Build history of the part. All positions in model axes, mm. A direction names the side the tool comes from. Give positions to 0.01 mm unless a question says otherwise; leave off trailing zeros. Order: outer loops, then holes, each group sorted by start corner. A loop starts at its lowest first (then second) coordinate and runs counter-clockwise, first axis right, second up. Notation, with made-up numbers: M -6.5,86.25 L -0.5,86.25 A19 cw -0.5,94.25 Z; hole C 47.25,15.25 d11. An arc over 180 degrees is marked long. One line per item, written item: value.
from build123d import *

# Parameters (mm, degrees)
F0_W     = 254
F0_H     = 127
F1_DEPTH = 76.2
F2_W     = 203.2
F2_H     = 76.2
F3_DEPTH = 152.401
F4_W     = 127
F4_H     = 55.738516
F5_DEPTH = 127.001
F6_R     = 25.4
F7_DEPTH = 254.001


with BuildPart() as f1:
    # F0 (on Top) → F1 (new body, symmetric)
    with BuildSketch(Plane.XY):
        Rectangle(F0_W, F0_H)
    extrude(amount=F1_DEPTH, both=True)

    # F2 (on face) → F3 (cut, through all)
    with BuildSketch(Plane.XY.offset(76.2)):
        Rectangle(F2_W, F2_H)
    extrude(amount=-F3_DEPTH, mode=Mode.SUBTRACT)

    # F4 (on face) → F5 (cut, through all)
    with BuildSketch(Plane.XZ.offset(63.5)):
        with Locations((0, 53.269258)):
            Rectangle(F4_W, F4_H)
    extrude(amount=-F5_DEPTH, mode=Mode.SUBTRACT)

    # F6 (on face) → F7 (cut, through all)
    with BuildSketch(Plane.YZ.offset(127)):
        Circle(F6_R)
    extrude(amount=-F7_DEPTH, mode=Mode.SUBTRACT)


solid = f1.part
1) Saw through at C-C, the plane y = -33. Write the cut outline in (x, z).
Check values:
outline: M -127,-76.2 L -101.6,-76.2 L -101.6,76.2 L -127,76.2 Z; M 101.6,-76.2 L 127,-76.2 L 127,76.2 L 101.6,76.2 Z
2) Saw through at B-B, the plane z = 45. Write the cut outline in (x, y).
Check values:
outline: M -127,-63.5 L -63.5,-63.5 L -63.5,-38.1 L -101.6,-38.1 L -101.6,38.1 L -63.5,38.1 L -63.5,63.5 L -127,63.5 Z; M 63.5,-63.5 L 127,-63.5 L 127,63.5 L 63.5,63.5 L 63.5,38.1 L 101.6,38.1 L 101.6,-38.1 L 63.5,-38.1 Z
3) Saw through at D-D, the plane y = 0. Write the cut outline in (x, z), then the cut area to 3 significant figures.
Check values:
outline: M -127,-76.2 L -101.6,-76.2 L -101.6,-25.4 L -127,-25.4 Z; M -127,25.4 L -101.6,25.4 L -101.6,76.2 L -127,76.2 Z; M 101.6,-76.2 L 127,-76.2 L 127,-25.4 L 101.6,-25.4 Z; M 101.6,25.4 L 127,25.4 L 127,76.2 L 101.6,76.2 Z
area: 5,160 mm^2
4) Tool access for faces 4 (the face through (-1, 38.1, -16)), 5 (the face through (63.5, 51, 50)), 6 (the face through (-2, 43, -76.2)): list every direction of +Z, -Z, +X, -X, +Y, -Y with a clear straight run to the whole face (end or side of a thin tool).
Check values:
face 4: +Z, -Z
face 5: +Z, +Y, -Y
face 6: -Z, +X, -X, +Y, -Y
5) Saw through at A-A, the plane x = -89. Write the cut outline in (y, z).
Check values:
outline: M -63.5,-76.2 L -38.1,-76.2 L -38.1,76.2 L -63.5,76.2 Z; M 38.1,-76.2 L 63.5,-76.2 L 63.5,76.2 L 38.1,76.2 Z
6) Pin check, flat tips, straight feed: pin 1 (4 mm diameter, centred on y = 9, z = -21.5, fed in from -X); pin 2 (20.5 mm diameter, centred on x = -2.5, y = -50, fed in from +Z). Stop position of each tip, or through.
Check values:
pin 1: through
pin 2: z = 25.4
7) Drill centre lines: probe 1 along X at (y, z) = (-36, -63); probe 2 along Y at (x, z) = (-31.5, -58.5); probe 3 along X at (y, z) = (-51, 56). Where is each one in solid material? Low to high. Write a range as from..to.
Check values:
probe 1: -127..-101.6, 101.6..127
probe 2: -63.5..-38.1, 38.1..63.5
probe 3: -127..-63.5, 63.5..127
8) Mould opens along Y. For faces 1 (the face through (-2, 63.5, -16)), 2 (the face through (101.6, -26, 1)), 3 (the face through (-103, 1, 76.2)) say: released by +Y, released by -Y, zero draft, split by the parting line, or undercut.
Check values:
face 1: released by +Y
face 2: undercut
face 3: zero draft
